The model under review builds one solid part; all positions refer to its coordinate system, in mm. A direction names the side the tool comes from. Coordinates: 2 decimals unless noted, no trailing zeros. Loops run counter-clockwise (first coordinate to the right, second up) from the corner with the lowest first, then second, coordinate; pieces in that order, holes last. Notation, with made-up numbers: (-34.5, 45) - (2.5, 45) arc R19 cw to (2.5, 70) - close; hole circle Ø7 at (21.25, 32). An arc over 180 degrees is marked (long way). One line per item, written item: value. Start each with the question number.
1. We need section C-C, the plane x = 39. Give the boundary of the cut face in (y, z) (3 decimals), then the cut area to 3 significant figures.
2. We need section B-B, the plane x = 16.5. Give the boundary of the cut face in (y, z) (3 decimals).
3. Insertion check: P1, Ø2, axis at x = 8.5, z = 8.5, coming from the -Y side; P2, Ø10, axis at x = 34, z = 3, coming from the +Y side (3 decimals); P3, Ø2, axis at x = 34.5, z = 6.5, coming from the -Y side (3 decimals). Each pin has a flat end and moves straight along its axis. Give the tip position at first contact, or say it passes through.
4. To check wall thickness, follow line 1 (X direction, y = 35.5, z = 5) (3 decimals); line 2 (Y direction, x = 41.3, z = 0); line 3 (Y direction, x = 29, z = -8.25) (3 decimals). State the ranges of each line that lie inside material, in increasing order.
5. Mouldability with a two-part tool opening along Z and no side actions: class faces 1 (the face through (27.541, -2.033, -4.877)), 2 (the face through (34.4, 4.02, 2.47)), 3 (the face through (40.64, 31, 0)), 4 (the face through (28.829, 43, 0)) as +Z half, -Z half, draft (parallel to the pull), parting line (faces both ways), or undercut.
6. We need section A-A, the plane y = 8. Give the boundary of the cut face in (x, z), then the cut area to 3 significant figures.
7. For faces 5 (the face through (16, 20, -9.906)), 6 (the face through (26.289, -3, 0)), 7 (the face through (26.289, 43, 0)), list the 3-axis set-ups (+Z, -Z, +X, -X, +Y, -Y) from which the entire face can be reached by the end or side of a thin tool; tool diameter is ignored.
Autodesk Inventor part; units mm, degrees
ref_plane "YZ Plane" through (0, 0, 0) normal (1, 0, 0) x (0, 1, 0)
ref_plane "XZ Plane" through (0, 0, 0) normal (0, 1, 0) x (-1, 0, 0)
ref_plane "XY Plane" through (0, 0, 0) normal (0, 0, 1) x (1, 0, 0)
sketch "Sketch1" plane through (0, 0, 0) normal (0, 0, 1) x (1, 0, 0)
  line L0 (0, 0) -> (33.02, 0)
  line L1 (33.02, 0) -> (33.02, 40.005)
  line L2 (33.02, 40.005) -> (0, 40.005)
  line L3 (0, 40.005) -> (0, 0)
  dimension "d0" = 33.02
  dimension "d1" = 40.005
extrude "Extrusion1" add sketch "Sketch1" along normal mid plane 19.812
ref_plane "Work Plane1" through (26.289, 0, 9.906) normal (-1, 0, 0) x (0, 0, 1)
sketch "Sketch2" plane through (26.289, 0, 9.906) normal (-1, 0, 0) x (0, 0, 1)
  line L0 (-19.812, 40.005) -> (0, 40.005)
  line L1 (-19.812, 0) -> (0, 0)
  line L2 (-9.906, 40.005) -> (0, 40.005)
  line L3 (0, 40.005) -> (0, 46.609)
  line L4 (-9.906, 46.609) -> (-9.906, 44.323)
  arc A0 (-6.7754, 46.609) -> (-3.1052, 46.609) centre (-4.9403, 44.6913) ccw
  line L5 (0, 44.6913) -> (-2.286, 44.6913)
  line L6 (-4.9403, 40.005) -> (-4.9403, 42.037)
  line L7 (-9.906, 40.005) -> (-9.2583, 40.005)
  line L8 (-9.2583, 40.005) -> (-9.2583, 44.323)
  line L9 (-9.2583, 44.323) -> (-9.906, 44.323)
  line L10 (-9.906, 44.323) -> (-9.906, 40.005)
  line L11 (0, 46.609) -> (-3.1052, 46.609)
  line L12 (-6.7754, 46.609) -> (-9.906, 46.609)
  line L13 (-9.906, 40.005) -> (-19.812, 40.005)
  line L14 (-19.812, 40.005) -> (-19.812, 46.609)
  arc A1 (-16.7068, 46.609) -> (-13.0366, 46.609) centre (-14.8717, 44.6913) ccw
  line L15 (-19.812, 44.6913) -> (-17.526, 44.6913)
  line L16 (-14.8717, 40.005) -> (-14.8717, 42.037)
  line L17 (-10.5537, 40.005) -> (-10.5537, 44.323)
  line L18 (-10.5537, 44.323) -> (-9.906, 44.323)
  line L19 (-19.812, 46.609) -> (-16.7068, 46.609)
  line L20 (-13.0366, 46.609) -> (-9.906, 46.609)
  line L21 (0, 0) -> (0, 40.005)
  line L22 (-19.812, 40.005) -> (-19.812, 0)
  line L23 (0, 20.0025) -> (-19.812, 20.0025) construction
  line L24 (-19.812, 0) -> (0, 0)
  line L25 (0, 0) -> (0, -6.604)
  arc A2 (-3.1052, -6.604) -> (-6.7754, -6.604) centre (-4.9403, -4.6863) ccw
  line L26 (-9.2583, 0) -> (-9.2583, -4.318)
  line L27 (-9.2583, -4.318) -> (-9.906, -4.318)
  line L28 (0, -6.604) -> (-3.1052, -6.604)
  line L29 (-6.7754, -6.604) -> (-9.906, -6.604)
  line L30 (-19.812, -6.604) -> (-16.7068, -6.604)
  line L31 (-19.812, 0) -> (-19.812, -6.604)
  arc A3 (-13.0366, -6.604) -> (-16.7068, -6.604) centre (-14.8717, -4.6863) ccw
  line L32 (-9.906, 0) -> (-19.812, 0)
  line L33 (-10.5537, 0) -> (-10.5537, -4.318)
  line L34 (-10.5537, -4.318) -> (-9.906, -4.318)
  line L35 (-13.0366, -6.604) -> (-9.906, -6.604)
  dimension "d5" = 6.604
  dimension "d6" = 2.286
  dimension "d7" = 2.032
  dimension "d8" = 0.6477
  dimension "d9" = 4.318
  dimension "d11" = 4.318
extrude "Extrusion2" add sketch "Sketch2" against normal blind 2.54 contours L14 L15 A1 L16 L0 | L16 A1 L20 L4 L18 L17 L0 | L14 L19 A1 L15 | L1 L33 L34 L27 L26 L25 L28 A2 L29 L35 A3 L30 L31 | L17 L18 L10 L0 | L1 L26 L27 L34 L33 | L10 L9 L8 L0 | L8 L9 L4 L12 A0 L6 L0 | L6 A0 L5 L3 L0 | L5 A0 L11 L3
fillet "Fillet1" radius 1.27 4 edges at (27.559, 46.609, 9.906) (27.559, 46.609, -9.906) (27.559, -6.604, 9.906) (27.559, -6.604, -9.906)
sketch "Sketch3" plane through (33.02, 0, 9.906) normal (1, 0, 0) x (0, 0, -1)
  line L0 (1.016, 5.715) -> (18.796, 5.715)
  line L1 (18.796, 5.715) -> (18.796, 31.115)
  line L2 (9.906, 40.005) -> (9.906, 40.005)
  line L3 (1.016, 31.115) -> (1.016, 5.715)
  line L4 (19.812, 40.005) -> (0, 40.005) construction
  line L5 (0, 0) -> (0, 40.005) construction
  arc A0 (9.906, 40.005) -> (1.016, 31.115) centre (9.906, 31.115) ccw
  arc A1 (18.796, 31.115) -> (9.906, 40.005) centre (9.906, 31.115) ccw
  line L6 (9.906, 5.715) -> (9.906, 3.429) construction
  arc A2 (5.461, 5.715) -> (9.906, 3.429) centre (9.906, 8.8935) ccw
  arc A3 (9.906, 3.429) -> (14.351, 5.715) centre (9.906, 8.8935) ccw
  point P0 (9.906, 0)
  point P1 (18.796, 40.005)
  point P2 (1.016, 40.005)
  dimension "d15" = 17.78
  dimension "d16" = 34.29
  dimension "d17" = 1.016
  dimension "d18" = 8.89
  dimension "d19" = 2.286
  dimension "d20" = 8.89
  dimension "d21" = 4.445
extrude "Extrusion3" add sketch "Sketch3" along normal blind 2.794
sketch "Sketch4" plane through (35.814, 0, 9.906) normal (1, 0, 0) x (0, 0, -1)
  arc A0 (18.796, 31.115) -> (1.016, 31.115) centre (9.906, 31.115) ccw
  circle A1 centre (9.906, 31.115) radius 4.445
  point P0 (9.906, 0)
  dimension "d24" = 8.89
extrude "Extrusion4" add sketch "Sketch4" along normal blind 4.826
sketch "Sketch5" plane through (40.64, 31.115, 0) normal (1, 0, 0) x (0, 0, -1)
  circle A0 centre (0, 0) radius 11.8745
  circle A1 centre (0, 0) radius 2.9845
  point P0 (0, -31.115)
  dimension "d27" = 23.749
  dimension "d28" = 5.969
extrude "Extrusion5" add sketch "Sketch5" along normal blind 1.905
properties part number "HS-322HD"
Findings below:
1. outline: circle Ø8.89 at (31.115, 0)
1. area: 62.1 mm2
2. outline: (0, -9.906) - (40.005, -9.906) - (40.005, 9.906) - (0, 9.906) - close
3. P1: y = 0
3. P2: y = 40.005
3. P3: y = 5.715
4. line 1: 0 to 35.814, 40.64 to 42.545
4. line 2: 19.24 to 28.13, 34.1 to 42.99
4. line 3: 0 to 40.005
5. face 1: undercut
5. face 2: +Z half
5. face 3: undercut
5. face 4: draft
6. outline: (0, -9.91) - (33.02, -9.91) - (33.02, -8.89) - (35.81, -8.89) - (35.81, 8.89) - (33.02, 8.89) - (33.02, 9.91) - (0, 9.91) - close
6. area: 704 mm2
7. face 5: -Z, -X, +Y, -Y
7. face 6: +Z, -Z, -X, -Y
7. face 7: +Z, -Z, -X, +Y
